from build123d import *

# Parameters (mm, degrees)
SKETCH_1_R      = 1.5
SKETCH_1_R_2    = 3
EXTRUDE_1_DEPTH = 2


with BuildPart() as part:
    # 草图1 → 凸台-拉伸1 (new body)
    with BuildSketch(Plane.XY):
        with BuildLine():
            Line((-38.6, -4), (-33.6, -4))
            Line((-33.6, -4), (-26, -4))
            Line((-26, -4), (-26, 1.1))
            Line((-26, 1.1), (-11, 1.1))
            Line((-11, 1.1), (-11, 4.1))
            Line((-11, 4.1), (11, 4.1))
            Line((11, 4.1), (11, 1.1))
            Line((11, 1.1), (26, 1.1))
            Line((26, 1.1), (26, -4))
            Line((26, -4), (33.6, -4))
            Line((33.6, -4), (38.6, -4))
            Line((38.6, -4), (41.6, 0))
            Line((41.6, 0), (43.145657482, 6.5))
            Line((43.145657482, 6.5), (43.145657482, 30.7))
            Line((43.145657482, 30.7), (41.6, 32.877506789))
            Line((41.6, 32.877506789), (15, 52.1))
            ThreePointArc((15, 52.1), (0, 67.1), (-15, 52.1))
            Line((-15, 52.1), (-41.6, 32.877506789))
            Line((-41.6, 32.877506789), (-43.145657482, 30.7))
            Line((-43.145657482, 30.7), (-43.145657482, 6.5))
            Line((-43.145657482, 6.5), (-41.6, 0))
            Line((-41.6, 0), (-38.6, -4))
        make_face()
        with BuildLine():
            Line((-30, -1.1), (-37.2, -1.1))
            ThreePointArc((-37.2, -1.1), (-37.655634919, 0), (-37.2, 1.1))
            Line((-37.2, 1.1), (-30, 1.1))
            ThreePointArc((-30, 1.1), (-29.544365081, 0), (-30, -1.1))
        make_face(mode=Mode.SUBTRACT)
        with BuildLine():
            Line((-40.2, 6.5), (-40.2, 11.7))
            ThreePointArc((-40.2, 11.7), (-39.1, 12.155634919), (-38, 11.7))
            Line((-38, 11.7), (-38, 6.5))
            Line((-38, 6.5), (-40.2, 6.5))
        make_face(mode=Mode.SUBTRACT)
        with Locations((-19.55, 11.6)):
            Circle(SKETCH_1_R, mode=Mode.SUBTRACT)
        with BuildLine():
            Line((-38, 30.7), (-38, 25.5))
            ThreePointArc((-38, 25.5), (-39.1, 25.044365081), (-40.2, 25.5))
            Line((-40.2, 25.5), (-40.2, 30.7))
            ThreePointArc((-40.2, 30.7), (-39.1, 31.155634919), (-38, 30.7))
        make_face(mode=Mode.SUBTRACT)
        with Locations((-19.55, 25.85)):
            Circle(SKETCH_1_R, mode=Mode.SUBTRACT)
        with Locations((19.55, 11.6)):
            Circle(SKETCH_1_R, mode=Mode.SUBTRACT)
        with BuildLine():
            Line((30, 1.1), (37.2, 1.1))
            ThreePointArc((37.2, 1.1), (37.655634919, 0), (37.2, -1.1))
            Line((37.2, -1.1), (30, -1.1))
            Line((30, -1.1), (30, 1.1))
        make_face(mode=Mode.SUBTRACT)
        with BuildLine():
            Line((38, 6.5), (38, 11.7))
            ThreePointArc((38, 11.7), (39.1, 12.155634919), (40.2, 11.7))
            Line((40.2, 11.7), (40.2, 6.5))
            Line((40.2, 6.5), (38, 6.5))
        make_face(mode=Mode.SUBTRACT)
        with Locations((0, 14.1)):
            Circle(SKETCH_1_R_2, mode=Mode.SUBTRACT)
        with Locations((19.55, 25.85)):
            Circle(SKETCH_1_R, mode=Mode.SUBTRACT)
        with BuildLine():
            Line((40.2, 30.7), (40.2, 25.5))
            ThreePointArc((40.2, 25.5), (39.1, 25.044365081), (38, 25.5))
            Line((38, 25.5), (38, 30.7))
            ThreePointArc((38, 30.7), (39.1, 31.155634919), (40.2, 30.7))
        make_face(mode=Mode.SUBTRACT)
        with Locations((-19.55, 40.1)):
            Circle(SKETCH_1_R, mode=Mode.SUBTRACT)
        with Locations((0, 33.1)):
            Circle(SKETCH_1_R_2, mode=Mode.SUBTRACT)
        with Locations((0, 52.1)):
            Circle(SKETCH_1_R_2, mode=Mode.SUBTRACT)
        with Locations((19.55, 40.1)):
            Circle(SKETCH_1_R, mode=Mode.SUBTRACT)
    extrude(amount=EXTRUDE_1_DEPTH)


solid = part.part
Could you check a few things on this model? Use its own coordinates, in mm. A direction names the side the tool comes from. Give positions to 0.01 mm unless a question says otherwise; leave off trailing zeros. Write each loop counter-clockwise with the first axis right and the second up, starting at its lowest first coordinate (ties: lowest second). Pieces come first, ordered by that corner, then holes. Notation, with made-up numbers: (40, 7) -> (87, 7) arc R25 cw to (87, 19) -> close; hole circle Ø9 at (-13, -30). An arc over 180 degrees is marked (long way). Answer as a JSON object with one key per item and string values.
Q1. We'd pull the mould along Y, two halves only. Please class faces 1 (the flat face through (39, 6.5, 1)), 2 (the flat face through (-1, 24, 2)), 3 (the flat face through (40.1, -2, 1)): released by +Y, released by -Y, zero draft, split by the parting line, or undercut.
Taken from the geometry:
{"face 1": "undercut", "face 2": "zero draft", "face 3": "released by -Y"}
Q2. Suppose I cut it at C-C on x = -19.55. Write out the boundary of the cut face in (y, z).
Taken from the geometry:
{"outline": "(1.1, 0) -> (10.1, 0) -> (10.1, 2) -> (1.1, 2) -> close; (13.1, 0) -> (24.35, 0) -> (24.35, 2) -> (13.1, 2) -> close; (27.35, 0) -> (38.6, 0) -> (38.6, 2) -> (27.35, 2) -> close; (41.6, 0) -> (48.81, 0) -> (48.81, 2) -> (41.6, 2) -> close"}
Q3. Suppose I cut it at D-D on y = 40.1. Write out the boundary of the cut face in (x, z).
Taken from the geometry:
{"outline": "(-31.61, 0) -> (-21.05, 0) -> (-21.05, 2) -> (-31.61, 2) -> close; (-18.05, 0) -> (18.05, 0) -> (18.05, 2) -> (-18.05, 2) -> close; (21.05, 0) -> (31.61, 0) -> (31.61, 2) -> (21.05, 2) -> close"}
Q4. Suppose I cut it at A-A on y = 7.5. Write out the boundary of the cut face in (x, z).
Taken from the geometry:
{"outline": "(-43.15, 0) -> (-40.2, 0) -> (-40.2, 2) -> (-43.15, 2) -> close; (-38, 0) -> (38, 0) -> (38, 2) -> (-38, 2) -> close; (40.2, 0) -> (43.15, 0) -> (43.15, 2) -> (40.2, 2) -> close"}
Q5. Will these pins go through, and if not, where does the flat tip stop? pin 1 Ø1 at (x, z) = (-18.5, 1) entering from -Y; pin 2 Ø1 at (y, z) = (2.5, 1) entering from -X; pin 3 Ø0.6 at (x, z) = (-39.5, 0.5) entering from +Y.
Taken from the geometry:
{"pin 1": "stops at y = 1.1", "pin 2": "stops at x = -42.31", "pin 3": "stops at y = 34.61"}
Q6. Which directions (+Z, -Z, +X, -X, +Y, -Y) give clear straight access to the entire face, cutting with the end or side of a thin tool? Please do faces 4 (the flat face through (34, 1.1, 1)), 5 (the flat face through (-1, 24, 0)), 6 (the flat face through (11, 3, 1)).
Taken from the geometry:
{"face 4": "+Z, -Z", "face 5": "-Z, +X, -X, +Y, -Y", "face 6": "+Z, -Z, -Y"}
Q7. Suppose I cut it at B-B on y = 15.5. Write out the boundary of the cut face in (x, z), then the cut area to 3 significant figures.
Taken from the geometry:
{"outline": "(-43.15, 0) -> (-2.65, 0) -> (-2.65, 2) -> (-43.15, 2) -> close; (2.65, 0) -> (43.15, 0) -> (43.15, 2) -> (2.65, 2) -> close", "area": "162 mm²"}
Q8. Please list where these lines run through material, in increasing order: L1, parallel to X at y = 29, z = 0.55; L2, parallel to X at y = -0.5, z = 1.3 (3 decimals); L3, parallel to Y at x = -19.55, z = 0.6.
Taken from the geometry:
{"L1": "x = -43.15 to -40.2, -38 to 38, 40.2 to 43.15", "L2": "x = -41.225 to -37.573, -29.627 to -26, 26 to 30, 37.573 to 41.225", "L3": "y = 1.1 to 10.1, 13.1 to 24.35, 27.35 to 38.6, 41.6 to 48.81"}
